from build123d import *

# Parameters (mm, degrees)
SCHIZZO2_R               = 10
SCHIZZO2_R_2             = 9.05
TAGLIO_ESTRUSIONE1_DEPTH = 1.2
TAGLIO_ESTRUSIONE2_START = -1.2
SCHIZZO3_R               = 10
SCHIZZO3_R_2             = 9.05
TAGLIO_ESTRUSIONE2_DEPTH = 1.2
SMUSSO1_SIZE             = 0.5
TAGLIO_ESTRUSIONE5_START = 9
TAGLIO_ESTRUSIONE5_DEPTH = 3.0000001


with BuildPart() as part:
    # Schizzo1 → Rivoluzione1 (revolve)
    with BuildSketch(Plane.XY, mode=Mode.PRIVATE) as rivoluzione1_sk:
        Polygon((-25, 0), (25, 0), (25, -10), (9, -10), (9, -12), (-6, -12), (-6, -15), (-11, -15), (-11, -10), (-25, -10), align=None)
    revolve(rivoluzione1_sk.sketch.rotate(Axis((-25, 0, 0), (1, 0, 0)), 270), axis=Axis((-25, 0, 0), (1, 0, 0)))

    # Schizzo2 → Taglio-Estrusione1 (cut)
    with BuildSketch(Plane.ZY.offset(23.2)):
        Circle(SCHIZZO2_R)
        Circle(SCHIZZO2_R_2, mode=Mode.SUBTRACT)
    extrude(amount=-TAGLIO_ESTRUSIONE1_DEPTH, mode=Mode.SUBTRACT)

    # Schizzo3 → Taglio-Estrusione2 (cut)
    with BuildSketch(Plane(origin=(22.2, 0, 0), x_dir=(0, 0, -1), z_dir=(1, 0, 0)).offset(TAGLIO_ESTRUSIONE2_START)):
        with Locations(Location((0, 0, 0), (0, 0, 180))):
            Circle(SCHIZZO3_R)
        with Locations(Location((0, 0, 0), (0, 0, 180))):
            Circle(SCHIZZO3_R_2, mode=Mode.SUBTRACT)
    extrude(amount=TAGLIO_ESTRUSIONE2_DEPTH, mode=Mode.SUBTRACT)

    # Smusso1
    smusso1_edges = [part.edges().sort_by_distance(p)[0] for p in [
        (-6, 0, -15),
        (-11, 0, -15),
        (-25, 0, -10),
        (25, 0, -10),
        (9, 0, -12),
    ]]
    chamfer(smusso1_edges, length=SMUSSO1_SIZE)

    # Taglio-Estrusione5: read off the stored shape, not the designer's step
    # Taglio-Estrusione5 outline → Taglio-Estrusione5 (cut)
    with BuildSketch(Plane(origin=(0, 0, 0), x_dir=(1, 0, 0), z_dir=(0, 1, 0)).offset(TAGLIO_ESTRUSIONE5_START)):
        with BuildLine():
            Line((3.5, 4), (-1.5, 4))
            ThreePointArc((-1.5, 4), (-5.5, 0), (-1.5, -4))
            Line((-1.5, -4), (3.5, -4))
            ThreePointArc((3.5, -4), (7.5, 0), (3.5, 4))
        make_face()
    extrude(amount=TAGLIO_ESTRUSIONE5_DEPTH, mode=Mode.SUBTRACT)


solid = part.part
Design review of the part built by this model. Coordinates are the model's own, in mm. A direction names the side the tool comes from. Coordinates: 2 decimals unless noted, no trailing zeros. Order: outer loops, then holes, each group sorted by start corner. A loop starts at its lowest first (then second) coordinate and runs counter-clockwise, first axis right, second up.
Item 1: For line 1 (X direction, y = -2.25, z = 9); line 2 (Y direction, x = 10, z = 0); line 3 (Z direction, x = 11, y = 0.5), list the stretches that pass through material, from the lowest coordinate up.
Item 2: The part is to be moulded in two halves that separate along X. For faces 1 (the flat face through (1, 10, -4)), 2 (the flat face through (22.2, 9, -2)), 3 (the cylindrical face through (14.92, 9.76, -2.17)), 4 (the flat face through (9, -5, 9)), say which applies: pulls with the +X half, pulls with the -X half, needs draft (parallel to the pull), parting line crosses it, or undercut.
Item 3: For faces 5 (the cylindrical face through (-23.86, 9.76, -2.17)), 6 (the cylindrical face through (-22.61, 2.72, 8.63)), 7 (the cylindrical face through (1.15, -10.12, 6.45)), 8 (the cylindrical face through (7.5, 10.5, 0.1)), list the 3-axis set-ups (+Z, -Z, +X, -X, +Y, -Y) from which the entire face can be reached by the end or side of a thin tool; tool diameter is ignored.
Item 4: For pin 1 Ø2.5 at (x, y) = (0, 10.5) entering from -Z; pin 2 Ø1.5 at (y, z) = (3.5, 11.5) entering from +X; pin 3 Ø10 at (y, z) = (11.5, 4) entering from +X; pin 4 Ø0.7 at (x, y) = (1.5, 10) entering from +Z, all flat-tipped, find the tip position at first contact; note any pin that passes through.
Item 5: Take a section at A-A, the plane x = 2. Write out the cut boundary in (y, z).
The answers:
1. line 1: x = -25 to -23.2, -22 to 21, 22.2 to 25
1. line 2: y = -10 to 10
1. line 3: z = -9.99 to 9.99
2. face 1: undercut
2. face 2: undercut
2. face 3: needs draft
2. face 4: pulls with the +X half
3. face 5: -X
3. face 6: none
3. face 7: +X
3. face 8: +Y
4. pin 1: stops at z = -7.64
4. pin 2: stops at x = 9
4. pin 3: stops at x = 25
4. pin 4: stops at z = 7.13
5. outline: (9, -4) - (9, 4) - (11.31, 4) arc R12 ccw (long way) to (11.31, -4) - close
